from build123d import *

# Parameters (mm, degrees)
SKETCH1_R           = 1.75
SKETCH1_R_2         = 2
BOSS_EXTRUDE1_DEPTH = 5


with BuildPart() as part:
    # Sketch1 → Boss-Extrude1 (new body)
    with BuildSketch(Plane.XY):
        Polygon((-72.5, 30), (72.5, 30), (72.5, -30), (25, -30), (25, -80), (-25, -80), (-25, -30), (-72.5, -30), align=None)
        with Locations((-11.5, -66.5)):
            Circle(SKETCH1_R, mode=Mode.SUBTRACT)
        with Locations((11.5, -66.5)):
            Circle(SKETCH1_R, mode=Mode.SUBTRACT)
        with Locations((11.5, -43.5)):
            Circle(SKETCH1_R, mode=Mode.SUBTRACT)
        with Locations((-11.5, -43.5)):
            Circle(SKETCH1_R, mode=Mode.SUBTRACT)
        with Locations((-63, 9)):
            Circle(SKETCH1_R_2, mode=Mode.SUBTRACT)
        with Locations((-39, 9)):
            Circle(SKETCH1_R_2, mode=Mode.SUBTRACT)
        with Locations((-39, -9)):
            Circle(SKETCH1_R_2, mode=Mode.SUBTRACT)
        with Locations((-63, -9)):
            Circle(SKETCH1_R_2, mode=Mode.SUBTRACT)
        with Locations((63, -9)):
            Circle(SKETCH1_R_2, mode=Mode.SUBTRACT)
        with Locations((39, -9)):
            Circle(SKETCH1_R_2, mode=Mode.SUBTRACT)
        with Locations((39, 9)):
            Circle(SKETCH1_R_2, mode=Mode.SUBTRACT)
        with Locations((63, 9)):
            Circle(SKETCH1_R_2, mode=Mode.SUBTRACT)
    extrude(amount=BOSS_EXTRUDE1_DEPTH)


solid = part.part
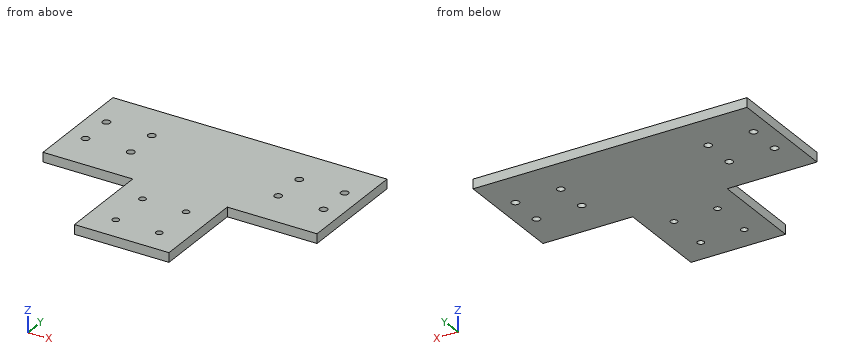
Model file for the job. Use its own axes, mm. Coordinates: 2 decimals unless noted, no trailing zeros. Write each loop counter-clockwise with the first axis right and the second up, starting at its lowest first coordinate (ties: lowest second). Pieces come first, ordered by that corner, then holes. Notation, with made-up numbers: (-24.75, -19) -> (-12.75, -19) arc R16 ccw to (-12.75, -5) -> close; hole circle Ø9 at (49.5, 8). An arc over 180 degrees is marked (long way). One line per item, written item: value. Start each with the question number.
1) Slice it at A-A on y = -9. Write the cut outline in (x, z).
2) Probe probe 1 along Y at (x, z) = (-63, 1.65); probe 2 along X at (y, z) = (-66.5, 3.85); probe 3 along Y at (x, z) = (-38.5, 1.05). List the from-to ranges inside material, lowest first.
3) Flat gauge pins, fed straight in: pin 1 Ø2 at (x, y) = (-11.5, -43.5) entering from +Z; pin 2 Ø2.5 at (x, z) = (-50, 3) entering from -Y; pin 3 Ø2.5 at (y, z) = (-43, 3) entering from -X. Where does each tip first touch, or does it go through?
4) Slice it at C-C on y = -43.5. Write the cut outline in (x, z), then the cut area to 3 significant figures.
5) Slice it at B-B on x = -39. Write the cut outline in (y, z), then the cut area to 3 significant figures.
6) Slice it at D-D on z = 1.85. Count the separate pieces of the cut face and the enclosed holes in it, then the cut area to 3 significant figures.
Answers follow:
1. outline: (-72.5, 0) -> (-65, 0) -> (-65, 5) -> (-72.5, 5) -> close; (-61, 0) -> (-41, 0) -> (-41, 5) -> (-61, 5) -> close; (-37, 0) -> (37, 0) -> (37, 5) -> (-37, 5) -> close; (41, 0) -> (61, 0) -> (61, 5) -> (41, 5) -> close; (65, 0) -> (72.5, 0) -> (72.5, 5) -> (65, 5) -> close
2. probe 1: -30 to -11, -7 to 7, 11 to 30
2. probe 2: -25 to -13.25, -9.75 to 9.75, 13.25 to 25
2. probe 3: -30 to -10.94, -7.06 to 7.06, 10.94 to 30
3. pin 1: through
3. pin 2: y = -30
3. pin 3: x = -25
4. outline: (-25, 0) -> (-13.25, 0) -> (-13.25, 5) -> (-25, 5) -> close; (-9.75, 0) -> (9.75, 0) -> (9.75, 5) -> (-9.75, 5) -> close; (13.25, 0) -> (25, 0) -> (25, 5) -> (13.25, 5) -> close
4. area: 215 mm2
5. outline: (-30, 0) -> (-11, 0) -> (-11, 5) -> (-30, 5) -> close; (-7, 0) -> (7, 0) -> (7, 5) -> (-7, 5) -> close; (11, 0) -> (30, 0) -> (30, 5) -> (11, 5) -> close
5. area: 260 mm2
6. separate pieces: 1
6. enclosed holes: 12
6. area: 11,100 mm2
